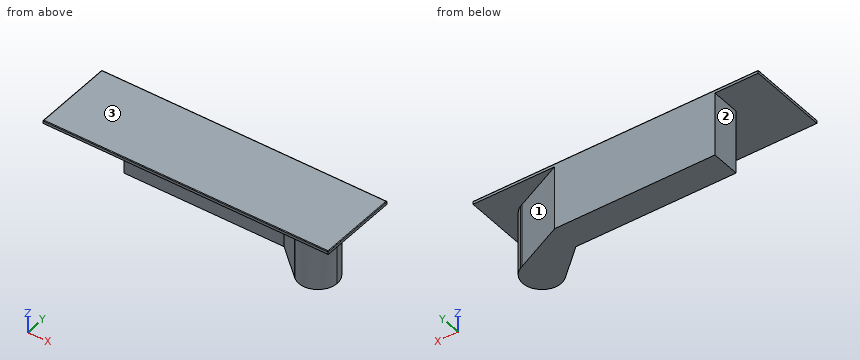
from build123d import *

# Parameters (mm, degrees)
F0_W     = 2260.6
F0_H     = 635
F1_DEPTH = 25.4
F2_R     = 5.08
F3_W     = 1270
F3_H     = 228.6
F4_DEPTH = 508


with BuildPart() as f1:
    # F0 (on Top) → F1 (new body)
    with BuildSketch(Plane.XY):
        with Locations((1130.3, 317.5)):
            Rectangle(F0_W, F0_H)
    extrude(amount=F1_DEPTH)

    # F2
    f2_edges = [f1.edges().sort_by_distance(p)[0] for p in [
        (0, 317.5, 25.4),
        (1130.3, 0, 25.4),
        (2260.6, 317.5, 25.4),
        (1130.3, 635, 25.4),
    ]]
    fillet(f2_edges, radius=F2_R)

    # F3 (on face) → F4 (join)
    with BuildSketch(Plane(origin=(0, 0, 0), x_dir=(1, 0, 0), z_dir=(0, 0, -1))):
        with Locations((977.9, -520.7)):
            Rectangle(F3_W, F3_H)
        with BuildLine():
            Line((1612.9, -406.4), (1612.9, -635))
            Line((1612.9, -635), (2012.596362, -446.22112))
            ThreePointArc((2012.596362, -446.22112), (1827.078225, -386.38716), (1852.147463, -193.077524))
            Line((1852.147463, -193.077524), (1612.9, -406.4))
        make_face()
        with BuildLine():
            Line((2028.944765, -438.499676), (2012.596362, -446.22112))
            ThreePointArc((2012.596362, -446.22112), (2020.88517, -442.60305), (2028.944765, -438.499676))
        make_face()
        with BuildLine():
            ThreePointArc((1852.147463, -193.077524), (1827.078225, -386.38716), (2012.596362, -446.22112))
            Line((2012.596362, -446.22112), (2028.944765, -438.499676))
            ThreePointArc((2028.944765, -438.499676), (2086.897334, -382.512605), (2108.2, -304.8))
            ThreePointArc((2108.2, -304.8), (2019.496552, -166.349614), (1856.64476, -189.067557))
            Line((1856.64476, -189.067557), (1852.147463, -193.077524))
        make_face()
        with BuildLine():
            ThreePointArc((1856.64476, -189.067557), (1854.376292, -191.050313), (1852.147463, -193.077524))
            Line((1852.147463, -193.077524), (1856.64476, -189.067557))
        make_face()
    extrude(amount=F4_DEPTH)


solid = f1.part
Build history of the part. All positions in model axes, mm. Face numbers are marked on the shaded views. A direction names the side the tool comes from. Round coordinates to 2 decimals unless told otherwise and drop trailing zeros. Write each loop counter-clockwise with the first axis right and the second up, starting at its lowest first coordinate (ties: lowest second). Pieces come first, ordered by that corner, then holes. Notation, with made-up numbers: M 18,74 L 54,74 A20 cw 54,112 Z; hole C 87.5,77.25 d9. An arc over 180 degrees is marked long. Use CSV: the item, a comma, the result in double quotes.
1. Saw through at A-A (z = -393). Give the cut face in (x, y).
Reply:
outline,"M 342.9,406.4 L 1612.9,406.4 L 1852.15,193.08 A152.4 ccw 1856.64,189.07 A152.4 ccw 2108.2,304.8 A152.4 ccw 2028.94,438.5 A152.4 ccw 2012.6,446.22 L 1612.9,635 L 342.9,635 Z"
2. Flat gauge pins, fed straight in: pin 1 (2 mm diameter, centred on y = 491.5, z = -373, fed in from -X); pin 2 (10 mm diameter, centred on x = 663.5, y = 91, fed in from -Z); pin 3 (5 mm diameter, centred on y = 372.5, z = -332.5, fed in from +X). Where does each tip first touch, or does it go through?
Reply:
pin 1,"stops at x = 342.9"
pin 2,"stops at z = 0"
pin 3,"stops at x = 2093.55"
3. Saw through at B-B (x = 1373). Give the cut face in (y, z).
Reply:
outline,"M 0,0 L 406.4,0 L 406.4,-508 L 635,-508 L 635,20.32 A5.08 ccw 629.92,25.4 L 5.08,25.4 A5.08 ccw 0,20.32 Z"
4. Saw through at D-D (x = 1658.5). Give the cut face in (y, z).
Reply:
outline,"M 0,0 L 365.74,0 L 365.74,-508 L 613.46,-508 L 613.46,0 L 635,0 L 635,20.32 A5.08 ccw 629.92,25.4 L 5.08,25.4 A5.08 ccw 0,20.32 Z"
5. Tool access for the marked faces 1, 2 and 3: list every direction of +Z, -Z, +X, -X, +Y, -Y with a clear straight run to the whole face (end or side of a thin tool).
Reply:
face 1,"-Z, +X, +Y"
face 2,"-Z, -X, +Y, -Y"
face 3,"+Z, +X, -X, +Y, -Y"
6. Saw through at C-C (y = 106). Give the cut face in (x, z).
Reply:
outline,"M 0,0 L 2260.6,0 L 2260.6,20.32 A5.08 ccw 2255.52,25.4 L 5.08,25.4 A5.08 ccw 0,20.32 Z"
7. Wall check: probe 1 along Z at (x, y) = (1150, 218); probe 2 along Y at (x, z) = (891, -426); probe 3 along X at (y, z) = (343, -314). Give the ranges that are in metal, low to high. Write a range as from..to.
Reply:
probe 1,"z = 0..25.4"
probe 2,"y = 406.4..635"
probe 3,"x = 1684..2103.33"
